Could you check a few things on this model? Use its own coordinates, in mm. Face numbers are marked on the shaded views. A direction names the side the tool comes from. Give positions to 0.01 mm unless a question says otherwise; leave off trailing zeros. Order: outer loops, then holes, each group sorted by start corner. A loop starts at its lowest first (then second) coordinate and runs counter-clockwise, first axis right, second up. Notation, with made-up numbers: (76, 21.25) -> (120, 21.25) arc R25 cw to (120, 50.25) -> close; hole circle Ø8 at (15, 44.5). An arc over 180 degrees is marked (long way). One line per item, written item: value.
```python
from build123d import *

# Parameters (mm, degrees)
F0_R     = 12.630129
F1_DEPTH = 6.35
F2_R     = 6.581493
F3_DEPTH = 15.24
F4_R     = 12.475408
F5_DEPTH = 6.35
F6_R     = 3.570848
F7_DEPTH = 27.941
F8_SIZE  = 2.54


with BuildPart() as f1:
    # F0 (on Top) → F1 (new body)
    with BuildSketch(Plane.XY):
        Circle(F0_R)
    extrude(amount=F1_DEPTH)

    # F2 (on face) → F3 (join)
    with BuildSketch(Plane.XY.offset(6.35)):
        Circle(F2_R)
    extrude(amount=F3_DEPTH)

    # F4 (on face) → F5 (join)
    with BuildSketch(Plane.XY.offset(21.59)):
        Circle(F4_R)
    extrude(amount=F5_DEPTH)

    # F6 (on face) → F7 (cut, through all)
    with BuildSketch(Plane.XY.offset(27.94)):
        Circle(F6_R)
    extrude(amount=-F7_DEPTH, mode=Mode.SUBTRACT)

    # F8
    f8_edges = [f1.edges().sort_by_distance(p)[0] for p in [
        (-3.570848, 0, 27.94),
        (-3.570848, 0, 0),
    ]]
    chamfer(f8_edges, length=F8_SIZE)


solid = f1.part
```
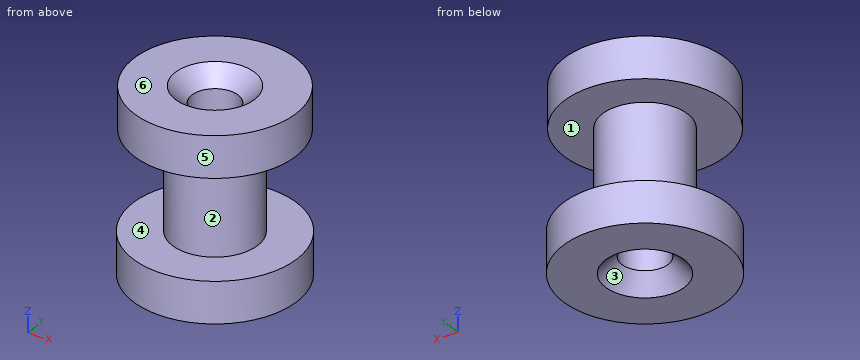
1) If I drill on line 1 along Z through (x, y) = (1, 9); line 2 along Y through (x, z) = (0, 15.5); line 3 along Y through (x, z) = (-2.75, 2.25), over which ranges is the centre line in solid material (lowest first)?
Answer below:
line 1: z = 0 to 6.35, 21.59 to 27.94
line 2: y = -6.58 to -3.57, 3.57 to 6.58
line 3: y = -12.33 to -2.71, 2.71 to 12.33
2) For P1, Ø3, axis at y = -1.5, z = 12, coming from the -X side; P2, Ø11.5, axis at x = 0, y = 0, coming from the +Z side; P3, Ø12, axis at y = 6.5, z = 24, coming from the -X side, each with a flat end and sliding along its axis, tell me the tip position at first contact or that it passes through.
Answer below:
P1: stops at x = -6.58
P2: stops at z = 27.58
P3: stops at x = -12.47
3) Suppose I cut it at D-D, the plane x = 8. Write out the boundary of the cut face in (y, z), then the cut area to 3 significant figures.
Answer below:
outline: (-9.77, 0) -> (9.77, 0) -> (9.77, 6.35) -> (-9.77, 6.35) -> close; (-9.57, 21.59) -> (9.57, 21.59) -> (9.57, 27.94) -> (-9.57, 27.94) -> close
area: 246 mm2
4) We'd pull the mould along Y, two halves only. Please class the marked faces 1, 2 and 3: +Y half, -Y half, draft (parallel to the pull), parting line (faces both ways), or undercut.
Answer below:
face 1: draft
face 2: parting line
face 3: undercut
5) Suppose I cut it at C-C, the plane z = 14.25. Write out the boundary of the cut face in (x, y).
Answer below:
outline: circle Ø13.16 at (0, 0); hole circle Ø7.14 at (0, 0)
6) Suppose I cut it at A-A, the plane y = 0. Write out the boundary of the cut face in (x, z), then the cut area to 3 significant figures.
Answer below:
outline: (-12.63, 0) -> (-6.11, 0) -> (-3.57, 2.54) -> (-3.57, 25.4) -> (-6.11, 27.94) -> (-12.48, 27.94) -> (-12.48, 21.59) -> (-6.58, 21.59) -> (-6.58, 6.35) -> (-12.63, 6.35) -> close; (3.57, 2.54) -> (6.11, 0) -> (12.63, 0) -> (12.63, 6.35) -> (6.58, 6.35) -> (6.58, 21.59) -> (12.48, 21.59) -> (12.48, 27.94) -> (6.11, 27.94) -> (3.57, 25.4) -> close
area: 307 mm2
7) For the marked faces 4, 5 and 6, which set-ups out of +Z, -Z, +X, -X, +Y, -Y let a thin tool reach every point of the face, with its end or its side?
Answer below:
face 4: none
face 5: +Z
face 6: +Z, +X, -X, +Y, -Y
